Work out the finished part from the listing and answer in its coordinate system (mm). Coordinates: 2 decimals unless noted, no trailing zeros. Write each question's results on one line, items separated by ' | '.
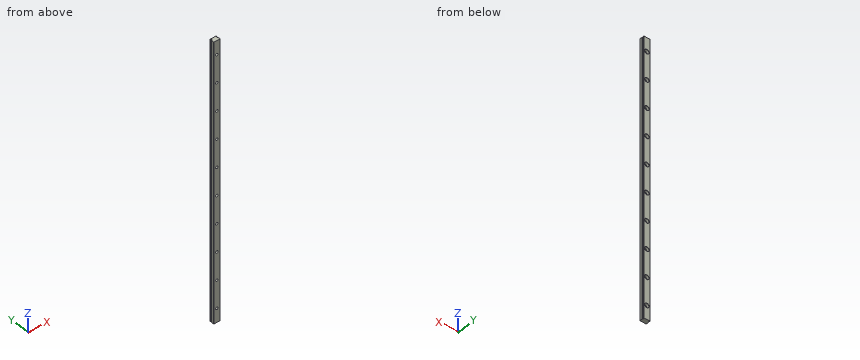
Autodesk Inventor part; units mm, degrees
ref_plane "YZ Plane" through (0, 0, 0) normal (1, 0, 0) x (0, 1, 0)
ref_plane "XZ Plane" through (0, 0, 0) normal (0, 1, 0) x (-1, 0, 0)
ref_plane "XY Plane" through (0, 0, 0) normal (0, 0, 1) x (1, 0, 0)
sketch "Skizze1" plane through (0, 0, 0) normal (0, 0, 1) x (1, 0, 0)
  arc A0 (-3.6501, 1.7625) -> (-4.5, 2.445) centre (-4.6, 1.45) ccw
  line L0 (-3.6501, 1.7625) -> (-3.1501, 1.7625)
  line L1 (-3.1501, 1.7625) -> (-3.1501, 1.2625)
  line L2 (-3.1501, 1.2625) -> (-3.6177, 1.2625)
  arc A1 (-4.5, 0.455) -> (-3.6177, 1.2625) centre (-4.6, 1.45) ccw
  line L3 (-4.5, 0.455) -> (-4.5, -3.05)
  line L4 (-4.5, -3.05) -> (-4.3, -3.25)
  line L5 (-4.3, -3.25) -> (4.3, -3.25)
  line L6 (4.3, -3.25) -> (4.5, -3.05)
  line L7 (4.5, -3.05) -> (4.5, 0.455)
  arc A2 (3.6177, 1.2625) -> (4.5, 0.455) centre (4.6, 1.45) ccw
  line L8 (3.6177, 1.2625) -> (3.1501, 1.2625)
  line L9 (3.1501, 1.2625) -> (3.1501, 1.7625)
  line L10 (3.1501, 1.7625) -> (3.6501, 1.7625)
  arc A3 (4.5, 2.445) -> (3.6501, 1.7625) centre (4.6, 1.45) ccw
  line L11 (4.5, 2.445) -> (4.5, 3.05)
  line L12 (4.5, 3.05) -> (4.3, 3.25)
  line L13 (4.3, 3.25) -> (-4.3, 3.25)
  line L14 (-4.3, 3.25) -> (-4.5, 3.05)
  line L15 (-4.5, 3.05) -> (-4.5, 2.445)
  circle A4 centre (-4.6, 1.45) radius 1 construction
  circle A5 centre (4.6, 1.45) radius 1 construction
  line L16 (0, -4.55) -> (0, 4.55) construction
  point P0 (0, 0)
  point P1 (0, 0)
  point P2 (0, 3.25)
  point P3 (0, -3.25)
  dimension "d0" = 9
  dimension "d1" = 6.5
  dimension "d2" = 4.7
  dimension "d4" = 2
  dimension "d5" = 6.3002
  dimension "d6" = 0.5
  dimension "d7" = 0.4499
  dimension "d8" = 3.25
  dimension "d12" = 0.2
  dimension "d13" = 0.2
  dimension "d18" = 1.4875
extrude "Extrusion1" add sketch "Skizze1" along normal mid plane 400
sketch "Skizze2" plane through (-4.3, 3.25, 200) normal (0, 1, 0) x (1, 0, 0)
  line L0 (0, 400) -> (0, 0)
  line L1 (8.6, 0) -> (0, 0)
  line L2 (8.6, 400) -> (8.6, 0)
  line L3 (0, 400) -> (8.6, 400)
  line L4 (8.6, 0) -> (0, 0)
  line L5 (4.3, 0) -> (4.3, 400) construction
  line L6 (0, 400) -> (8.6, 400)
  line L7 (0, 400) -> (0, 0)
  line L8 (0, 200) -> (8.6, 200) construction
  line L9 (8.6, 400) -> (8.6, 0)
  point P0 (4.3, 20)
  point P1 (4.3, 60)
  point P2 (4.3, 100)
  point P3 (4.3, 140)
  point P4 (4.3, 180)
  point P5 (4.3, 220)
  point P6 (4.3, 260)
  point P7 (4.3, 300)
  point P8 (4.3, 340)
  point P9 (4.3, 380)
  dimension "d23" = 40
  dimension "d28" = 20
hole "Bohrung1" at (0, 3.25, 180) at (0, 3.25, 140) at (0, 3.25, 100) at (0, 3.25, 60) at (0, 3.25, 20) at (0, 3.25, -20) at (0, 3.25, -60) at (0, 3.25, -100) at (0, 3.25, -140) at (0, 3.25, -180) direction (0, -1, 0) diameter 3.4 end through all counterbore diameter 6 counterbore depth 3.4
chamfer "Fase1" distance 0.25 angle 45 10 edges at (0, 3.25, 177) (0, 3.25, 137) (0, 3.25, 97) (0, 3.25, 57) (0, 3.25, 17) (0, 3.25, -23) (0, 3.25, -63) (0, 3.25, -103) (0, 3.25, -143) (0, 3.25, -183)
properties part number "Linear-Rail MGN9h (400mm)" material "Stahl, hochfest, niedrig legiert"
1) Find section B-B, the plane y = -1.5. Give the number of separate pieces and of enclosed holes in the cut face, and give its area (3 significant figures).
Check result:
separate pieces: 1 | enclosed holes: 10 | area: 3,510 mm^2
2) Given pin 1 Ø2 at (x, z) = (0, 100) entering from +Y; pin 2 Ø5 at (x, z) = (1, 178.5) entering from +Y; pin 3 Ø4.5 at (x, z) = (0, 180) entering from +Y, each flat-ended and moving along its own axis, determine where each tip first touches the part or whether it passes through.
Check result:
pin 1: through | pin 2: y = 3.25 | pin 3: y = -0.15
3) Straight lines are drawn through the part: probe 1 along X at (y, z) = (1.85, 60); probe 2 along X at (y, z) = (1.5, 60); probe 3 along Y at (x, z) = (3.5, -131). For each, find the intervals that lie inside material, in ascending order. Write a range as [from, to].
Check result:
probe 1: [-3.68, -3], [3, 3.68] | probe 2: [-3.15, -3], [3, 3.15] | probe 3: [-3.25, 1.26], [1.76, 3.25]
